Autodesk Inventor part; units mm, degrees
ref_plane "YZ Plane" through (0, 0, 0) normal (1, 0, 0) x (0, 1, 0)
ref_plane "XZ Plane" through (0, 0, 0) normal (0, 1, 0) x (-1, 0, 0)
ref_plane "XY Plane" through (0, 0, 0) normal (0, 0, 1) x (1, 0, 0)
sketch "Boceto1" plane through (0, 0, 0) normal (0, 1, 0) x (-1, 0, 0)
  line L0 (-25, 40) -> (25, 40)
  line L1 (25, 40) -> (25, -40)
  line L2 (25, -40) -> (-25, -40)
  line L3 (-25, -40) -> (-25, 40)
  line L4 (-25, 40) -> (25, -40) construction
  line L5 (25, 40) -> (-25, -40) construction
  point P0 (0, 0)
  dimension "d0" = 50
  dimension "d1" = 80
extrude "Extrusión1" add sketch "Boceto1" along normal blind 50
sketch "Boceto2" plane through (0, 0, 0) normal (0, -1, 0) x (1, 0, 0)
  line L0 (-25, 40) -> (25, 40)
  line L1 (21, 40) -> (11, 40)
  line L2 (11, 40) -> (11, 36)
  line L3 (11, 36) -> (21, 36)
  line L4 (21, 36) -> (21, 40)
  line L5 (-25, -40) -> (25, -40)
  line L6 (21, -40) -> (11, -40)
  line L7 (11, -40) -> (11, -36)
  line L8 (11, -36) -> (21, -36)
  line L9 (21, -36) -> (21, -40)
  line L10 (25, 40) -> (-25, 40)
  line L11 (-11, 40) -> (-11, 36)
  line L12 (-11, 36) -> (-21, 36)
  line L13 (-21, 36) -> (-21, 40)
  line L14 (-21, -36) -> (-21, -40)
  line L15 (-11, -40) -> (-11, -36)
  line L16 (-11, -36) -> (-21, -36)
  line L17 (25, -40) -> (-25, -40)
  point P0 (0, 0)
  dimension "d6" = 4
extrude "Extrusión2" add sketch "Boceto2" along normal blind 20
properties part number "Caja"
Input: part model. Units: mm. Frame: model coordinates. A direction names the side the tool comes from. Give positions to 0.01 mm unless a question says otherwise; leave off trailing zeros. Order: outer loops, then holes, each group sorted by start corner. A loop starts at its lowest first (then second) coordinate and runs counter-clockwise, first axis right, second up. Notation, with made-up numbers: (81.25, -22) - (89.25, -22) arc R25 cw to (89.25, -8) - close; hole circle Ø8 at (67.5, 77.5). An arc over 180 degrees is marked (long way). Answer as a JSON object with one key per item and string values. Group by question number.
Q1. Cut plane C-C, the plane z = -17. Output: boundary loops of the cut face in (x, y).
Q2. Cut plane B-B, the plane x = 17. Output: boundary loops of the cut face in (y, z), then the cut area to 3 significant figures.
Q3. Line query: probe 1 along Z at (x, y) = (11.5, -8); probe 2 along Y at (x, z) = (12, -8). Output: solid intervals per line, ascending.
Q4. Cut plane D-D, the plane x = 0.5. Output: boundary loops of the cut face in (y, z).
Q5. First-contact query: pin 1 Ø1.5 at (x, z) = (-8, -30.5) entering from -Y; pin 2 Ø1.2 at (y, z) = (-10.5, 37) entering from -X; pin 3 Ø10 at (x, y) = (-9.5, -3) entering from -Z; pin 4 Ø4.5 at (y, z) = (-8.5, -37) entering from +X. Flat tips, straight axial feed; report the tip coordinate or a pass-through.
Q6. Mould query, pull axis X, two halves, no side actions, for faces 4 (the face through (21, -10, -38)), 5 (the face through (-11, -10, 38)), 6 (the face through (-16, -10, -36)). Classes: pulls with the +X half, pulls with the -X half, needs draft (parallel to the pull), parting line crosses it, or undercut.
Q7. Set-up query: faces 1 (the face through (-21, -10, 38)), 2 (the face through (-11, -10, -38)), 3 (the face through (-16, -10, 36)). Return all of +Z, -Z, +X, -X, +Y, -Y with unobstructed straight access to the full face (end or side cutting, diameter ignored); none if empty.
Q8. Cut plane A-A, the plane y = -5. Output: boundary loops of the cut face in (x, z).
Results:
{
 "1": {"outline": "(-25, 0) - (25, 0) - (25, 50) - (-25, 50) - close"},
 "2": {"outline": "(-20, -40) - (50, -40) - (50, 40) - (-20, 40) - (-20, 36) - (0, 36) - (0, -36) - (-20, -36) - close", "area": "4,160 mm^2"},
 "3": {"probe 1": "-40 to -36, 36 to 40", "probe 2": "0 to 50"},
 "4": {"outline": "(0, -40) - (50, -40) - (50, 40) - (0, 40) - close"},
 "5": {"pin 1": "y = 0", "pin 2": "x = -21", "pin 3": "z = -40", "pin 4": "x = 21"},
 "6": {"face 4": "pulls with the +X half", "face 5": "undercut", "face 6": "needs draft"},
 "7": {"face 1": "+Z, -Z, -X, -Y", "face 2": "+Z, -Z, -Y", "face 3": "+X, -X, -Y"},
 "8": {"outline": "(-21, -40) - (-11, -40) - (-11, -36) - (-21, -36) - close; (-21, 36) - (-11, 36) - (-11, 40) - (-21, 40) - close; (11, -40) - (21, -40) - (21, -36) - (11, -36) - close; (11, 36) - (21, 36) - (21, 40) - (11, 40) - close"}
}
